```python
from build123d import *

# Parameters (mm, degrees)
F0_R     = 3.175
F1_DEPTH = 3.048


with BuildPart() as f1:
    # F0 (on Front) → F1 (new body)
    with BuildSketch(Plane.XZ):
        with BuildLine():
            ThreePointArc((0, -2.8766015808), (-3.2635982736, 0.2971620124), (0, 3.4709256057))
            Line((0, 3.4709256057), (0, 15.8749901004))
            ThreePointArc((0, 15.8749901004), (-10.4918952223, 11.913601197), (-15.7476019291, 2.0065322858))
            ThreePointArc((-15.7476019291, 2.0065322858), (-11.9135847518, -10.4919245087), (0, -15.8750098992))
            Line((0, -15.8750098992), (0, -2.8766015808))
        make_face()
        with BuildLine():
            Line((0, 15.8749901004), (0, 3.4709256057))
            ThreePointArc((0, 3.4709256057), (2.1875744482, 2.5106801941), (3.0864017264, 0.2971620124))
            ThreePointArc((3.0864017264, 0.2971620124), (2.1875744482, -1.9163561693), (0, -2.8766015808))
            Line((0, -2.8766015808), (0, -15.8750098992))
            ThreePointArc((0, -15.8750098992), (11.2253703753, -11.2253575191), (15.8750776924, -9.8994e-06))
            ThreePointArc((15.8750776924, -9.8994e-06), (15.8431590584, 1.0061699208), (15.747531509, 2.0083036452))
            ThreePointArc((15.747531509, 2.0083036452), (10.491322233, 11.9142426155), (0, 15.8749901004))
        make_face()
        with BuildLine():
            ThreePointArc((-15.7476019291, 2.0065322858), (-10.4918952223, 11.913601197), (0, 15.8749901004))
            Line((0, 15.8749901004), (0, 41.275))
            ThreePointArc((0, 41.275), (-6.7504945807, 44.0801452459), (-9.5249014384, 50.8433311461))
            Line((-9.5249014384, 50.8433311461), (-15.7476019291, 2.0065322858))
        make_face()
        with Locations((-5.4904264398, 36.6574451327)):
            Circle(F0_R, mode=Mode.SUBTRACT)
        with BuildLine():
            Line((0, 41.275), (0, 15.8749901004))
            ThreePointArc((0, 15.8749901004), (10.491322233, 11.9142426155), (15.747531509, 2.0083036452))
            Line((15.747531509, 2.0083036452), (9.525, 50.8))
            ThreePointArc((9.525, 50.8), (6.7351920908, 44.0648079092), (0, 41.275))
        make_face()
        with BuildLine():
            ThreePointArc((15.8750776924, -9.8994e-06), (11.2253703753, -11.2253575191), (0, -15.8750098992))
            Line((0, -15.8750098992), (0, -54.2240571164))
            ThreePointArc((0, -54.2240571164), (6.2034967284, -57.1581140139), (8.8250504044, -63.5))
            Line((8.8250504044, -63.5), (36.5125, -63.5))
            ThreePointArc((36.5125, -63.5), (37.3509047062, -59.9494011406), (39.6890045065, -57.1488718986))
            Line((39.6890045065, -57.1488718986), (18.2762879211, -56.5058330852))
            ThreePointArc((18.2762879211, -56.5058330852), (12.5071090556, -53.7661112831), (10.6150505702, -47.6661428387))
            Line((10.6150505702, -47.6661428387), (16.0036556786, 0))
            Line((16.0036556786, 0), (15.747531509, 2.0083036452))
            ThreePointArc((15.747531509, 2.0083036452), (15.8431590584, 1.0061699208), (15.8750776924, -9.8994e-06))
        make_face()
        with BuildLine():
            Line((0, -54.2240571164), (0, -15.8750098992))
            ThreePointArc((0, -15.8750098992), (-11.9135847518, -10.4919245087), (-15.7476019291, 2.0065322858))
            Line((-15.7476019291, 2.0065322858), (-16.0032708044, 0))
            Line((-16.0032708044, 0), (-10.1838874689, -64.5783643789))
            ThreePointArc((-10.1838874689, -64.5783643789), (-7.4881720596, -57.0444215396), (0, -54.2240571164))
        make_face()
        with BuildLine():
            ThreePointArc((-9.5249014384, 50.8433311461), (-6.7504945807, 44.0801452459), (0, 41.275))
            ThreePointArc((0, 41.275), (6.7351920908, 44.0648079092), (9.525, 50.8))
            ThreePointArc((9.525, 50.8), (0.0216656291, 60.3249753596), (-9.5249014384, 50.8433311461))
        make_face()
        with BuildLine():
            ThreePointArc((3.0864017264, 50.6975539029), (2.1875744482, 48.4840357212), (0, 47.5237903096))
            ThreePointArc((0, 47.5237903096), (-2.3647709953, 52.9110720846), (3.0864017264, 50.6975539029))
        make_face(mode=Mode.SUBTRACT)
        with BuildLine():
            Line((0, -60.598008398), (0, -54.2240571164))
            ThreePointArc((0, -54.2240571164), (-7.4881720596, -57.0444215396), (-10.1838874689, -64.5783643789))
            ThreePointArc((-10.1838874689, -64.5783643789), (-6.8613205089, -70.985095451), (0, -73.222937069))
            ThreePointArc((0, -73.222937069), (6.2800529577, -70.2074613128), (8.8276728625, -63.7234970927))
            ThreePointArc((8.8276728625, -63.7234970927), (8.8270172254, -63.6117408538), (8.8250504044, -63.5))
            Line((8.8250504044, -63.5), (2.6692960727, -63.5))
            ThreePointArc((2.6692960727, -63.5), (2.6757633798, -63.6168482324), (2.6779201256, -63.7338554285))
            ThreePointArc((2.6779201256, -63.7338554285), (-2.9115004676, -65.7956988268), (0, -60.598008398))
        make_face()
        with BuildLine():
            Line((36.5125, -63.5), (8.8250504044, -63.5))
            ThreePointArc((8.8250504044, -63.5), (8.8270172254, -63.6117408538), (8.8276728625, -63.7234970927))
            ThreePointArc((8.8276728625, -63.7234970927), (6.2800529577, -70.2074613128), (0, -73.222937069))
            Line((0, -73.222937069), (44.7674390348, -71.4311498983))
            ThreePointArc((44.7674390348, -71.4311498983), (38.9507166871, -69.2237915139), (36.5125, -63.5))
        make_face()
        with BuildLine():
            ThreePointArc((39.6890045065, -57.1488718986), (37.3509047062, -59.9494011406), (36.5125, -63.5))
            ThreePointArc((36.5125, -63.5), (38.9507166871, -69.2237915139), (44.7674390348, -71.4311498983))
            ThreePointArc((44.7674390348, -71.4311498983), (50.1737915139, -68.9992833129), (52.3875, -63.5))
            ThreePointArc((52.3875, -63.5), (48.0005988594, -56.4009047062), (39.6890045065, -57.1488718986))
        make_face()
        with BuildLine():
            ThreePointArc((47.3964347422, -63.4233355522), (44.2597697605, -66.5981041149), (41.0473604579, -63.5))
            ThreePointArc((41.0473604579, -63.5), (44.1830997239, -60.2485669896), (47.3964347422, -63.4233355522))
        make_face(mode=Mode.SUBTRACT)
        with BuildLine():
            ThreePointArc((8.8250504044, -63.5), (6.2034967284, -57.1581140139), (0, -54.2240571164))
            Line((0, -54.2240571164), (0, -60.598008398))
            ThreePointArc((0, -60.598008398), (1.8397162129, -61.5844347981), (2.6692960727, -63.5))
            Line((2.6692960727, -63.5), (8.8250504044, -63.5))
        make_face()
    extrude(amount=F1_DEPTH)


solid = f1.part
```
Here's how the part is built. I have some questions about the finished solid (model axes, mm). A direction names the side the tool comes from. Coordinates: 2 decimals unless noted, no trailing zeros. Order: outer loops, then holes, each group sorted by start corner. A loop starts at its lowest first (then second) coordinate and runs counter-clockwise, first axis right, second up. Notation, with made-up numbers: (49, -15.5) -> (103, -15.5) arc R16 cw to (103, 8.5) -> close; hole circle Ø9 at (16.5, 54). An arc over 180 degrees is marked (long way). Return JSON: item names as keys, results as strings.
1) If we section it at D-D on x = 24.5: List the corners of the cut face in (y, z) for me.
Conclusion:
{"outline": "(-3.05, -72.24) -> (0, -72.24) -> (0, -56.69) -> (-3.05, -56.69) -> close"}
2) On a 3-axis mill with a long thin cutter (end or side, diameter ignored), from which of +Z, -Z, +X, -X, +Y, -Y can I reach the whole of each face in a straight line? I mean faces 1 (the cylindrical face through (12.57, -1.5, -53.84)), 2 (the flat face through (13.27, -1.5, -24.17)), 3 (the flat face through (3, 0, -20)). Say none if no direction works.
Conclusion:
{"face 1": "+Y, -Y", "face 2": "+X, +Y, -Y", "face 3": "+Z, -Z, +X, -X, +Y"}
3) Thinking about a two-plate mould opening in X: for faces 4 (the cylindrical face through (-0.317, -1.503, 53.864)), 5 (the flat face through (22.07, -1.5, -72.34)), 6 (the flat face through (3, -3.048, -20)), which applies, +X half, -X half, draft (parallel to the pull), parting line (faces both ways), or undercut?
Conclusion:
{"face 4": "undercut", "face 5": "+X half", "face 6": "draft"}
4) If we section it at A-A on z = 49: List the corners of the cut face in (x, y) for me.
Conclusion:
{"outline": "(-9.76, -3.05) -> (-2.77, -3.05) -> (-2.77, 0) -> (-9.76, 0) -> close; (2.59, -3.05) -> (9.75, -3.05) -> (9.75, 0) -> (2.59, 0) -> close"}
5) I'm going to push flat-ended pins straight in: P1, Ø4, axis at x = -0.09, z = 50.7, coming from the -Y side; P2, Ø1, axis at x = 23.5, y = -1.5, coming from the -Z side. Where does each tip first touch, or does it pass through?
Conclusion:
{"P1": "passes through", "P2": "stops at z = -72.3"}
6) If I drill on probe 1 along X at (y, z) = (-2.55, -61); probe 2 along Z at (x, y) = (43.5, -0.15); probe 3 along Z at (x, y) = (47, -0.5), over which ranges is the centre line in solid material (lowest first)?
Conclusion:
{"probe 1": "x = -10.51 to -2.11, 1.12 to 42.17, 46.27 to 51.98", "probe 2": "z = -71.48 to -66.52, -60.33 to -55.62", "probe 3": "z = -71.02 to -64.96, -61.89 to -55.98"}
7) If we section it at C-C on z = -10: List the corners of the cut face in (x, y) for me, plus the area to 3 significant figures.
Conclusion:
{"outline": "(-15.1, -3.05) -> (14.87, -3.05) -> (14.87, 0) -> (-15.1, 0) -> close", "area": "91.4 mm²"}
8) If we section it at B-B on y = -2.4: State how many separate pieces and enclosed holes the cut face has, plus the area to 3 significant figures.
Conclusion:
{"separate pieces": "1", "enclosed holes": "5", "area": "3,730 mm²"}
